```python
from build123d import *

# Parameters (mm, degrees)
F0_W          = 66.080972
F0_H          = 105.729562
F1_DEPTH      = 6.35
F2_W          = 66.080972
F2_H          = 105.729562
F2_W_2        = 38.1
F2_H_2        = 101.6
F3_DEPTH      = 25.4
F4_W          = 38.1
F4_H          = 101.6
F4_W_2        = 25.4
F4_H_2        = 76.2
F5_DEPTH      = 19.05
F6_W          = 6.35
F6_H          = 48.527334
F7_DEPTH      = 25.4
F7_DEPTH_BACK = 25.4


with BuildPart() as f1:
    # F0 (on Top) → F1 (new body)
    with BuildSketch(Plane.XY):
        with Locations((0.146851, 2e-06)):
            Rectangle(F0_W, F0_H)
    extrude(amount=F1_DEPTH)

    # F2 (on face) → F3 (join)
    with BuildSketch(Plane.XY.offset(6.35)):
        with Locations((0.146851, 2e-06)):
            Rectangle(F2_W, F2_H)
        with Locations((-0.440535, 0.589116)):
            Rectangle(F2_W_2, F2_H_2, mode=Mode.SUBTRACT)
    extrude(amount=F3_DEPTH)

    # F4 (on face) → F5 (join)
    with BuildSketch(Plane.XY.offset(6.35)):
        with Locations((-0.440535, 0.589116)):
            Rectangle(F4_W, F4_H)
        with Locations((-0.128517, -1.191032)):
            Rectangle(F4_W_2, F4_H_2, mode=Mode.SUBTRACT)
    extrude(amount=F5_DEPTH)

    # F6 (on face) → F7 (cut, two sides)
    with BuildSketch(Plane.XY.offset(6.35)) as f7_sk:
        with Locations((-0.011918, -0.932903)):
            Rectangle(F6_W, F6_H)
    extrude(amount=F7_DEPTH, mode=Mode.SUBTRACT)
    extrude(f7_sk.sketch, amount=-F7_DEPTH_BACK, mode=Mode.SUBTRACT)


solid = f1.part
```
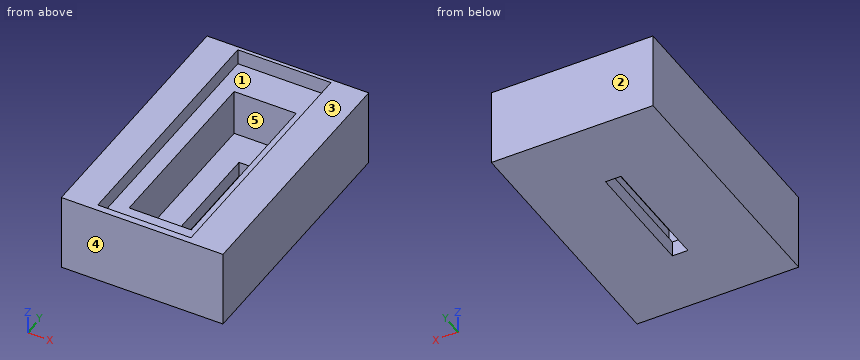
Here's how the part is built. I have some questions about the finished solid (model axes, mm). Face numbers are marked on the shaded views. A direction names the side the tool comes from. Round coordinates to 2 decimals unless told otherwise and drop trailing zeros. Write each loop counter-clockwise with the first axis right and the second up, starting at its lowest first coordinate (ties: lowest second). Pieces come first, ordered by that corner, then holes.
Q1. If we section it at D-D on z = 28: Write out the boundary of the cut face in (x, y).
Q2. If we section it at B-B on z = 15.5: Write out the boundary of the cut face in (x, y).
Q3. If we mould it in two halves opening along Y, with no side actions, what happens to the marked faces 3, 4 and 5? For each: +Y half, -Y half, draft (parallel to the pull), parting line (faces both ways), or undercut.
Q4. Will these pins go through, and if not, where does the flat tip stop? P1, Ø11.5, axis at x = -7, y = 16, coming from the +Z side; P2, Ø8, axis at x = 25.5, y = -12, coming from the -Z side; P3, Ø4, axis at x = -12.5, y = 8, coming from the +Z side.
Q5. Which directions (+Z, -Z, +X, -X, +Y, -Y) give clear straight access to the entire face, cutting with the end or side of a thin tool? Please do the marked faces 1 and 2.
Q6. Please list where these lines run through material, in increasing order: probe 1 along X at (y, z) = (-36.5, 11); probe 2 along Y at (x, z) = (4, 14); probe 3 along Z at (x, y) = (8, 44).
Q7. If we section it at C-C on x = -11.5: Write out the boundary of the cut face in (y, z).
Q8. If we section it at A-A on y = -17.5: Write out the boundary of the cut face in (x, z).
Answer below:
1. outline: (-32.89, -52.86) - (33.19, -52.86) - (33.19, 52.86) - (-32.89, 52.86) - close; hole (-19.49, -50.21) - (18.61, -50.21) - (18.61, 51.39) - (-19.49, 51.39) - close
2. outline: (-32.89, -52.86) - (33.19, -52.86) - (33.19, 52.86) - (-32.89, 52.86) - close; hole (-12.83, -39.29) - (12.57, -39.29) - (12.57, 36.91) - (-12.83, 36.91) - close
3. face 3: draft
3. face 4: -Y half
3. face 5: undercut
4. P1: stops at z = 6.35
4. P2: stops at z = 0
4. P3: stops at z = 25.4
5. face 1: +Z
5. face 2: +Z, -Z, +X, -X, +Y
6. probe 1: x = -32.89 to -12.83, 12.57 to 33.19
6. probe 2: y = -52.86 to -39.29, 36.91 to 52.86
6. probe 3: z = 0 to 25.4
7. outline: (-52.86, 0) - (52.86, 0) - (52.86, 31.75) - (51.39, 31.75) - (51.39, 25.4) - (36.91, 25.4) - (36.91, 6.35) - (-39.29, 6.35) - (-39.29, 25.4) - (-50.21, 25.4) - (-50.21, 31.75) - (-52.86, 31.75) - close
8. outline: (-32.89, 0) - (-3.19, 0) - (-3.19, 6.35) - (-12.83, 6.35) - (-12.83, 25.4) - (-19.49, 25.4) - (-19.49, 31.75) - (-32.89, 31.75) - close; (3.16, 0) - (33.19, 0) - (33.19, 31.75) - (18.61, 31.75) - (18.61, 25.4) - (12.57, 25.4) - (12.57, 6.35) - (3.16, 6.35) - close
